Read the model definition and answer for the solid it produces. Units are mm, in the model's axes. A direction names the side the tool comes from. Round coordinates to 2 decimals unless told otherwise and drop trailing zeros. Write each loop counter-clockwise with the first axis right and the second up, starting at its lowest first coordinate (ties: lowest second). Pieces come first, ordered by that corner, then holes.
from build123d import *

# Parameters (mm, degrees)
BOSS_EXTRUDE1_DEPTH      = 24
BOSS_EXTRUDE1_DEPTH_BACK = 3
SKETCH1_W                = 75
SKETCH1_H                = 24
CUT_EXTRUDE1_START       = -5
SKETCH2_W                = 30
SKETCH2_H                = 20
CUT_EXTRUDE1_DEPTH       = 20
CUT_EXTRUDE2_DEPTH       = 3
CUT_EXTRUDE3_REACH       = 63.438
SKETCH20_R               = 1
CUT_EXTRUDE4_REACH       = 63.438
SKETCH21_R               = 1.5
SKETCH24_W               = 75
SKETCH24_H               = 24
BOSS_EXTRUDE2_DEPTH      = 2
CUT_EXTRUDE5_DEPTH       = 5


with BuildPart() as part:
    # Sketch1 → Boss-Extrude1 (new, two sides: drawn at the far end of the back side and taken through both)
    with BuildSketch(Plane.XY.offset(-BOSS_EXTRUDE1_DEPTH_BACK)):
        with Locations((13.875, 8.15625)):
            Rectangle(SKETCH1_W, SKETCH1_H)
    extrude(amount=BOSS_EXTRUDE1_DEPTH + BOSS_EXTRUDE1_DEPTH_BACK)

    # Sketch2 → Cut-Extrude1 (cut)
    with BuildSketch(Plane.XY.offset(24).offset(CUT_EXTRUDE1_START)):
        with Locations((-3.625, 8.15625)):
            Rectangle(SKETCH2_W, SKETCH2_H)
        with Locations((31.375, 8.15625)):
            Rectangle(SKETCH2_W, SKETCH2_H)
    extrude(amount=-CUT_EXTRUDE1_DEPTH, mode=Mode.SUBTRACT)

    # Sketch3 → Cut-Extrude2 (cut)
    with BuildSketch(Plane.XY.offset(24)):
        with BuildLine():
            ThreePointArc((-8.784211185, 12.48145261), (13.902958167, -2.563657938), (36.582455444, 12.493015262))
            ThreePointArc((36.582455444, 12.493015262), (35.249734837, 15.767745141), (31.975004957, 14.435024533))
            ThreePointArc((31.975004957, 14.435024533), (13.901683811, 2.436341899), (-4.177751221, 14.425810242))
            ThreePointArc((-4.177751221, 14.425810242), (-7.453160019, 15.756861408), (-8.784211185, 12.48145261))
        make_face()
    extrude(amount=-CUT_EXTRUDE2_DEPTH, mode=Mode.SUBTRACT)

    # Sketch20 → Cut-Extrude3 (cut, up to next)
    with BuildSketch(Plane.XY.offset(24), mode=Mode.PRIVATE) as cut_extrude3_sk1:
        with Locations((27.875, 4.90625)):
            Circle(SKETCH20_R)
    cut_extrude3_tool1 = extrude(cut_extrude3_sk1.sketch, amount=-CUT_EXTRUDE3_REACH, mode=Mode.PRIVATE) & part.part
    # Sketch20 → Cut-Extrude3 (cut, up to next)
    with BuildSketch(Plane.XY.offset(24), mode=Mode.PRIVATE) as cut_extrude3_sk2:
        with Locations((-0.125, 4.90625)):
            Circle(SKETCH20_R)
    cut_extrude3_tool2 = extrude(cut_extrude3_sk2.sketch, amount=-CUT_EXTRUDE3_REACH, mode=Mode.PRIVATE) & part.part
    add(cut_extrude3_tool1.solids().sort_by_distance((27.875, 4.90625, 24))[0], mode=Mode.SUBTRACT)
    add(cut_extrude3_tool2.solids().sort_by_distance((-0.125, 4.90625, 24))[0], mode=Mode.SUBTRACT)

    # Sketch21 → Cut-Extrude4 (cut, up to next)
    with BuildSketch(Plane(origin=(0, 0, -3), x_dir=(-1, 0, 0), z_dir=(0, 0, -1)), mode=Mode.PRIVATE) as cut_extrude4_sk1:
        with Locations((-32.680205402, 5.075855595)):
            Circle(SKETCH21_R)
    cut_extrude4_tool1 = extrude(cut_extrude4_sk1.sketch, amount=-CUT_EXTRUDE4_REACH, mode=Mode.PRIVATE) & part.part
    # Sketch21 → Cut-Extrude4 (cut, up to next)
    with BuildSketch(Plane(origin=(0, 0, -3), x_dir=(-1, 0, 0), z_dir=(0, 0, -1)), mode=Mode.PRIVATE) as cut_extrude4_sk2:
        with Locations((-27.861682335, 5.087799818)):
            Circle(SKETCH21_R)
    cut_extrude4_tool2 = extrude(cut_extrude4_sk2.sketch, amount=-CUT_EXTRUDE4_REACH, mode=Mode.PRIVATE) & part.part
    # Sketch21 → Cut-Extrude4 (cut, up to next)
    with BuildSketch(Plane(origin=(0, 0, -3), x_dir=(-1, 0, 0), z_dir=(0, 0, -1)), mode=Mode.PRIVATE) as cut_extrude4_sk3:
        with Locations(Location((0.111682335, 5.087799818, 0), (0, 0, 180))):
            Circle(SKETCH21_R)
    cut_extrude4_tool3 = extrude(cut_extrude4_sk3.sketch, amount=-CUT_EXTRUDE4_REACH, mode=Mode.PRIVATE) & part.part
    # Sketch21 → Cut-Extrude4 (cut, up to next)
    with BuildSketch(Plane(origin=(0, 0, -3), x_dir=(-1, 0, 0), z_dir=(0, 0, -1)), mode=Mode.PRIVATE) as cut_extrude4_sk4:
        with Locations(Location((4.930205402, 5.075855595, 0), (0, 0, 180))):
            Circle(SKETCH21_R)
    cut_extrude4_tool4 = extrude(cut_extrude4_sk4.sketch, amount=-CUT_EXTRUDE4_REACH, mode=Mode.PRIVATE) & part.part
    add(cut_extrude4_tool1.solids().sort_by_distance((32.680205, 5.075856, -3))[0], mode=Mode.SUBTRACT)
    add(cut_extrude4_tool2.solids().sort_by_distance((27.861682, 5.0878, -3))[0], mode=Mode.SUBTRACT)
    add(cut_extrude4_tool3.solids().sort_by_distance((-0.111682, 5.0878, -3))[0], mode=Mode.SUBTRACT)
    add(cut_extrude4_tool4.solids().sort_by_distance((-4.930205, 5.075856, -3))[0], mode=Mode.SUBTRACT)

    # Sketch24 → Boss-Extrude2 (add)
    with BuildSketch(Plane.XY.offset(24)):
        with Locations((13.875, 8.15625)):
            Rectangle(SKETCH24_W, SKETCH24_H)
        with BuildLine():
            ThreePointArc((-7.862919192, 12.870324137), (13.902703295, -1.563657971), (35.660965347, 12.881417116))
            ThreePointArc((35.660965347, 12.881417116), (34.861332982, 14.846255044), (32.896495055, 14.046622679))
            ThreePointArc((32.896495055, 14.046622679), (13.901938682, 1.436341932), (-5.099043214, 14.036938715))
            ThreePointArc((-5.099043214, 14.036938715), (-7.064288492, 14.835569415), (-7.862919192, 12.870324137))
        make_face(mode=Mode.SUBTRACT)
    extrude(amount=BOSS_EXTRUDE2_DEPTH)

    # Sketch26 → Cut-Extrude5 (cut)
    with BuildSketch(Plane.XY.offset(26)):
        with BuildLine():
            Line((23.705970435, 5.064731747), (26.205970435, 0.734604728))
            ThreePointArc((26.205970435, 0.734604728), (13.896683604, -2.563658738), (1.587396774, 0.734604728))
            Line((1.587396774, 0.734604728), (4.087396774, 5.064731747))
            ThreePointArc((4.087396774, 5.064731747), (13.896683604, 2.436341262), (23.705970435, 5.064731747))
        make_face()
    extrude(amount=-CUT_EXTRUDE5_DEPTH, mode=Mode.SUBTRACT)


solid = part.part
Q1. Straight lines are drawn through the part: probe 1 along X at (y, z) = (2.5, 13.75) (3 decimals); probe 2 along Z at (x, y) = (33, 14.75); probe 3 along Z at (x, y) = (-18, -1.5). For each, find the intervals that lie inside material, in ascending order.
Verdict:
probe 1: x = -23.625 to -18.625, 11.375 to 16.375, 46.375 to 51.375
probe 2: z = -3 to -1, 19 to 21, 24 to 26
probe 3: z = -3 to -1, 19 to 26
Q2. Section C-C (z = 22.25) is taken. Determine the outline of the cut face in (x, y) (3 decimals), then the cut area to 3 significant figures.
Verdict:
outline: (-23.625, -3.844) - (51.375, -3.844) - (51.375, 20.156) - (-23.625, 20.156) - close; hole (-8.784, 12.481) arc R24.619 ccw to (36.582, 12.493) arc R2.5 ccw to (31.975, 14.435) arc R19.619 cw to (-4.178, 14.426) arc R2.5 ccw to start
area: 1,520 mm2
Q3. Section D-D (y = 9) is taken. Determine the outline of the cut face in (x, z) (3 decimals), then the cut area to 3 significant figures.
Verdict:
outline: (-23.625, -3) - (51.375, -3) - (51.375, 26) - (33.579, 26) - (33.579, 24) - (34.769, 24) - (34.769, 21) - (28.541, 21) - (28.541, 24) - (29.856, 24) - (29.856, 26) - (-2.062, 26) - (-2.062, 24) - (-0.748, 24) - (-0.748, 21) - (-6.975, 21) - (-6.975, 24) - (-5.786, 24) - (-5.786, 26) - (-23.625, 26) - close; hole (-18.625, -1) - (11.375, -1) - (11.375, 19) - (-18.625, 19) - close; hole (16.375, -1) - (46.375, -1) - (46.375, 19) - (16.375, 19) - close
area: 923 mm2
Q4. Section B-B (x = 41) is taken. Determine the outline of the cut face in (y, z).
Verdict:
outline: (-3.84, -3) - (20.16, -3) - (20.16, 26) - (-3.84, 26) - close; hole (-1.84, -1) - (18.16, -1) - (18.16, 19) - (-1.84, 19) - close
Q5. Flat-ended cylindrical pins translate along their axes: pin 1 Ø4 at (x, y) = (32.68, 5.08) entering from -Z; pin 2 Ø2.5 at (x, y) = (-0.11, 5.09) entering from -Z. Find the tip coordinate at first contact, or state that the pin passes through.
Verdict:
pin 1: stops at z = -3
pin 2: stops at z = 19
Q6. Which of the six approach directions +Z, -Z, +X, -X, +Y, -Y give full straight-line access (tool end or side, diameter ignored) to faces 1 (the cylindrical face through (-0.3, 3.6, -2)), 2 (the cylindrical face through (29.418, 8.482, 24.986)), 3 (the flat face through (12, 2, 21))?
Verdict:
face 1: -Z
face 2: +Z
face 3: none
Q7. Section A-A (z = 13.5) is taken. Determine the outline of the cut face in (x, y) (3 decimals), then the cut area to 3 significant figures.
Verdict:
outline: (-23.625, -3.844) - (51.375, -3.844) - (51.375, 20.156) - (-23.625, 20.156) - close; hole (-18.625, -1.844) - (11.375, -1.844) - (11.375, 18.156) - (-18.625, 18.156) - close; hole (16.375, -1.844) - (46.375, -1.844) - (46.375, 18.156) - (16.375, 18.156) - close
area: 600 mm2
Q8. Determine the mould class of faces 4 (the cylindrical face through (33.786, 6.09, -2.014)), 5 (the flat face through (-4, 18.156, 9)) for opening direction Z: pulls with the +Z half, pulls with the -Z half, needs draft (parallel to the pull), parting line crosses it, or undercut.
Verdict:
face 4: needs draft
face 5: undercut
